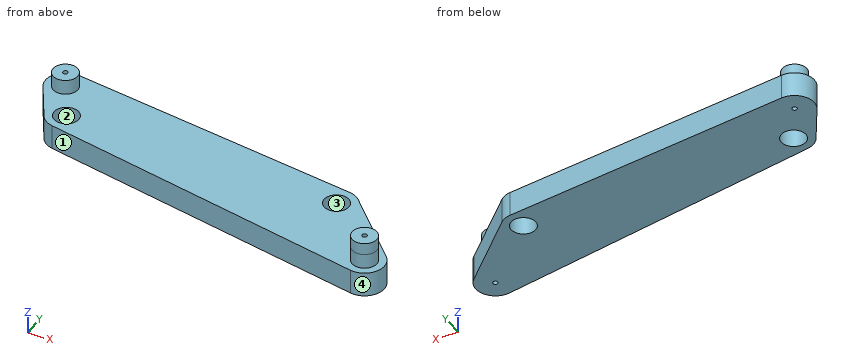
```python
from build123d import *

# Parameters (mm, degrees)
SKETCH2_R           = 2.5
BOSS_EXTRUDE1_DEPTH = 5
SKETCH4_R           = 2.5
SKETCH4_R_2         = 0.5
BOSS_EXTRUDE3_DEPTH = 8
SKETCH5_R           = 2.5
SKETCH5_R_2         = 0.5
BOSS_EXTRUDE4_DEPTH = 2.4


with BuildPart() as part:
    # Sketch2 → Boss-Extrude1 (new body)
    with BuildSketch(Plane.XY):
        with BuildLine():
            Line((-58.980456911, 11.76034449), (0.519543089, 3.966115855))
            ThreePointArc((0.519543089, 3.966115855), (1.767996055, 3.588062144), (2.828427125, 2.828427125))
            Line((2.828427125, 2.828427125), (15.556349186, -9.899494937))
            ThreePointArc((15.556349186, -9.899494937), (16.265540761, -14.594805544), (11.989145433, -16.659106246))
            Line((11.989145433, -16.659106246), (-55.738776628, -3.931184185))
            ThreePointArc((-55.738776628, -3.931184185), (-57.312663934, -3.263676689), (-58.464101615, -2))
            Line((-58.464101615, -2), (-62.964101615, 5.794228634))
            ThreePointArc((-62.964101615, 5.794228634), (-62.826595982, 10.015435327), (-58.980456911, 11.76034449))
        make_face()
        with Locations((-55, 0)):
            Circle(SKETCH2_R, mode=Mode.SUBTRACT)
        with Locations((-59.5, 7.794228634)):
            Circle(SKETCH2_R, mode=Mode.SUBTRACT)
        Circle(SKETCH2_R, mode=Mode.SUBTRACT)
        with Locations((12.727922061, -12.727922061)):
            Circle(SKETCH2_R, mode=Mode.SUBTRACT)
    extrude(amount=BOSS_EXTRUDE1_DEPTH)

    # Sketch4 → Boss-Extrude3 (add)
    # profile 1 of 2: a face of its own
    with BuildSketch(Plane(origin=(0, 0, 0), x_dir=(-1, 0, 0), z_dir=(0, 0, -1))):
        with Locations((59.5, 7.794228634)):
            Circle(SKETCH4_R)
        with Locations((59.5, 7.794228634)):
            Circle(SKETCH4_R_2, mode=Mode.SUBTRACT)
    # profile 2 of 2: a face of its own
    with BuildSketch(Plane(origin=(0, 0, 0), x_dir=(-1, 0, 0), z_dir=(0, 0, -1))):
        with Locations((-12.727922061, -12.727922061)):
            Circle(SKETCH4_R)
        with Locations((-12.727922061, -12.727922061)):
            Circle(SKETCH4_R_2, mode=Mode.SUBTRACT)
    extrude(amount=-BOSS_EXTRUDE3_DEPTH)

    # Sketch5 → Boss-Extrude4 (add)
    with BuildSketch(Plane.XY.offset(8)):
        with Locations((12.727922061, -12.727922061)):
            Circle(SKETCH5_R)
        with Locations(Location((12.727922061, -12.727922061, 0), (0, 0, 180))):
            Circle(SKETCH5_R_2, mode=Mode.SUBTRACT)
    extrude(amount=BOSS_EXTRUDE4_DEPTH)


solid = part.part
```
The model under review builds one solid part; all positions refer to its coordinate system, in mm. Face numbers are marked on the shaded views. Give positions to 0.01 mm unless a question says otherwise; leave off trailing zeros. Write each loop counter-clockwise with the first axis right and the second up, starting at its lowest first coordinate (ties: lowest second). Pieces come first, ordered by that corner, then holes. Notation, with made-up numbers: M 11.5,37 L 41.5,37 A13 ccw 41.5,44 Z; hole C 60.5,54.5 d8. An arc over 180 degrees is marked long. Write item = value, one per line. Start each with the question number.
Q1. We need section A-A (y = 0). State the section outline as (x, z) points, plus the area to 3 significant figures.
Q2. Clearance check with flat-ended pins moving along their axes: pin 1 (5 mm diameter, centred on x = -7.5, y = -9.5, fed in from +Z); pin 2 (1 mm diameter, centred on y = 1.5, z = 3, fed in from -X); pin 3 (6 mm diameter, centred on x = 5, z = 3, fed in from -Y). State where each tip first meets the part, or that it passes through.
Q3. We need section D-D (x = -55). State the section outline as (y, z) points.
Q4. Mouldability with a two-part tool opening along Y and no side actions: class the marked faces 1, 2, 3 and 4 as released by +Y, released by -Y, zero draft, split by the parting line, or undercut.
Q5. We need section C-C (z = 6.5). State the section outline as (x, y) points.
Q6. For line 1 (Z direction, x = -32, y = 7); line 2 (Y direction, x = -59.5, z = 2.5); line 3 (Y direction, x = -2, z = 3), list the stretches that pass through material, from the lowest coordinate up.
Q7. We need section B-B (x = -1). State the section outline as (y, z) points.
Result set:
q1.outline = M -59.62,0 L -57.5,0 L -57.5,5 L -59.62,5 Z; M -52.5,0 L -2.5,0 L -2.5,5 L -52.5,5 Z; M 2.5,0 L 5.66,0 L 5.66,5 L 2.5,5 Z
q1.area = 276 mm2
q2.pin_1 = 5
q2.pin_2 = -60.77
q2.pin_3 = -15.91
q3.outline = M -4.07,0 L -2.5,0 L -2.5,5 L -4.07,5 Z; M 2.5,0 L 11.24,0 L 11.24,5 L 2.5,5 Z
q4.face_1 = released by -Y
q4.face_2 = undercut
q4.face_3 = undercut
q4.face_4 = split by the parting line
q5.outline = C -59.5,7.79 d5; C 12.73,-12.73 d5; hole C -59.5,7.79 d1; hole C 12.73,-12.73 d1
q6.line_1 = 0 to 5
q6.line_2 = -0.21 to 7.29, 8.29 to 11.79
q6.line_3 = -14.03 to -1.5, 1.5 to 4.3
q7.outline = M -14.22,0 L -2.29,0 L -2.29,5 L -14.22,5 Z; M 2.29,0 L 4.17,0 L 4.17,5 L 2.29,5 Z
